Work out the finished part from the listing and answer in its coordinate system (mm). Coordinates: 2 decimals unless noted, no trailing zeros. Write each loop counter-clockwise with the first axis right and the second up, starting at its lowest first coordinate (ties: lowest second). Pieces come first, ordered by that corner, then holes. Notation, with made-up numbers: (-3.75, 39.5) - (6.25, 39.5) arc R16 ccw to (6.25, 59.5) - close; hole circle Ø7 at (71, 69.25). An arc over 180 degrees is marked (long way). Answer as a JSON object with one key per item and string values. Group by question number.
from build123d import *

# Parameters (mm, degrees)
SKETCH1_R           = 8.6
BOSS_EXTRUDE1_DEPTH = 2
FILLET1_R           = 1
SHELL1_T            = -0.2


with BuildPart() as part:
    # Sketch1 → Boss-Extrude1 (new body)
    with BuildSketch(Plane(origin=(0, 0, 0), x_dir=(1, 0, 0), z_dir=(0, 1, 0))):
        with Locations(Location((0, 0, 0), (0, 0, 270))):
            Circle(SKETCH1_R)
    extrude(amount=BOSS_EXTRUDE1_DEPTH)

    # Fillet1
    fillet1_edges = [part.edges().sort_by_distance(p)[0] for p in [
        (0, 2, -8.6),
    ]]
    fillet(fillet1_edges, radius=FILLET1_R)

    # Shell1
    shell1_openings = [part.faces().sort_by_distance(p)[0] for p in [
        (0, 0, 0),
    ]]
    offset(amount=SHELL1_T, openings=shell1_openings, kind=Kind.INTERSECTION)


solid = part.part
Q1. Section A-A on x = 0 is taken. Determine the outline of the cut face in (y, z), plus the area to 3 significant figures.
Q2. Section B-B on z = 0 is taken. Determine the outline of the cut face in (x, y), plus the area to 3 significant figures.
Q3. Section C-C on y = 0.45 is taken. Determine the outline of the cut face in (x, z).
Q4. For a pull along X with two mould halves and no side action, classify faces 1 (the face through (0, 1.8, 0)), 2 (the face through (0, 2, 0)), 3 (the face through (2.523, 0.493, 8.012)), 4 (the face through (-5.233, 0.493, -6.825)) as +X half, -X half, draft (parallel to the pull), parting line (faces both ways), or undercut.
Q5. Consider L1, parallel to X at y = 0.6, z = 0; L2, parallel to Z at x = -3.75, y = 0.7; L3, parallel to Y at x = -6, z = 4. Determine where each line is inside the solid, lowest interval first. Write a range as from..to.
Q6. Flat-ended cylindrical pins translate along their axes: pin 1 Ø8 at (x, z) = (5.5, -6) entering from +Y; pin 2 Ø4.5 at (x, z) = (3, 1) entering from -Y; pin 3 Ø1 at (x, y) = (0.5, 1.5) entering from +Z. Find the tip coordinate at first contact, or state that the pin passes through.
Numbers:
{
 "1": {"outline": "(0, -8.6) - (1, -8.6) arc R1 ccw to (2, -7.6) - (2, 7.6) arc R1 ccw to (1, 8.6) - (0, 8.6) - (0, 8.4) - (1, 8.4) arc R0.8 cw to (1.8, 7.6) - (1.8, -7.6) arc R0.8 cw to (1, -8.4) - (0, -8.4) - close", "area": "4.01 mm²"},
 "2": {"outline": "(-8.6, 0) - (-8.4, 0) - (-8.4, 1) arc R0.8 cw to (-7.6, 1.8) - (7.6, 1.8) arc R0.8 cw to (8.4, 1) - (8.4, 0) - (8.6, 0) - (8.6, 1) arc R1 ccw to (7.6, 2) - (-7.6, 2) arc R1 ccw to (-8.6, 1) - close", "area": "4.01 mm²"},
 "3": {"outline": "circle Ø17.2 at (0, 0); hole circle Ø16.8 at (0, 0)"},
 "4": {"face 1": "undercut", "face 2": "draft", "face 3": "undercut", "face 4": "parting line"},
 "5": {"L1": "x = -8.6..-8.4, 8.4..8.6", "L2": "z = -7.74..-7.52, 7.52..7.74", "L3": "y = 1.8..2"},
 "6": {"pin 1": "stops at y = 2", "pin 2": "stops at y = 1.8", "pin 3": "stops at z = 8.59"}
}
